Geometry: final body of the model. Coordinates: model frame, mm. Face numbers are marked on the shaded views. A direction names the side the tool comes from. Coordinates: 2 decimals unless noted, no trailing zeros. Order: outer loops, then holes, each group sorted by start corner. A loop starts at its lowest first (then second) coordinate and runs counter-clockwise, first axis right, second up. Notation, with made-up numbers: (-28, 68.5) -> (2, 68.5) arc R15 ccw to (2, 77.5) -> close; hole circle Ø10 at (64, 35). An arc over 180 degrees is marked (long way). Use one line per item in the form item = value.
Autodesk Inventor part; units mm, degrees
ref_plane "YZ Plane" through (0, 0, 0) normal (1, 0, 0) x (0, 1, 0)
ref_plane "XZ Plane" through (0, 0, 0) normal (0, 1, 0) x (-1, 0, 0)
ref_plane "XY Plane" through (0, 0, 0) normal (0, 0, 1) x (1, 0, 0)
sketch "Sketch1" plane through (0, 0, 0) normal (0, 0, 1) x (1, 0, 0)
  point P0 (0, 0)
sketch "Sketch2" plane through (0, 0, 0) normal (0, 1, 0) x (-1, 0, 0)
  arc A0 (-30.6952, -7.0747) -> (-30.6952, 7.0747) centre (0, 0) ccw
  line L0 (-30.6952, 7.0747) -> (-30.6952, -7.0747)
  dimension "d0" = 63
extrude "Extrusion1" add sketch "Sketch2" along normal blind 27
sketch "Sketch3" plane through (0, 27, 0) normal (0, 1, 0) x (0, 0, 1)
  point P0 (0, 0)
  point P1 (0, 0)
hole "Hole1" at (0, 27, 0) direction (0, -1, 0) diameter 58.5 depth 26
sketch "Sketch4" plane through (0, 0, 0) normal (0, -1, 0) x (0, 0, 1)
  circle A0 centre (0, 0) radius 30
  dimension "d11" = 60
extrude "Extrusion2" add sketch "Sketch4" along normal blind 5
sketch "Sketch5" plane through (0, -5, 0) normal (0, -1, 0) x (1, 0, 0)
  point P0 (0, 0)
  point P1 (0, 0)
hole "Hole2" at (0, -5, 0) direction (0, 1, 0) diameter 51.8 depth 11
sketch "Sketch6" plane through (30.6952, 0, 7.0747) normal (1, 0, 0) x (0, 0, -1)
  circle A0 centre (6.9063, 13.867) radius 6.5
  point P0 (7.0747, 0)
  dimension "d23" = 13
extrude "Extrusion3" add sketch "Sketch6" along normal blind 5
sketch "Sketch7" plane through (35.6952, 13.867, 0.1684) normal (1, 0, 0) x (0, 0, -1)
  point P0 (0.1684, -13.867)
  point P1 (0.2284, -0.2272)
hole "Hole3" at (35.6952, 13.6397, -0.06) direction (-1, 0, 0) diameter 4.1 depth 10
properties part number "microscope_holder"
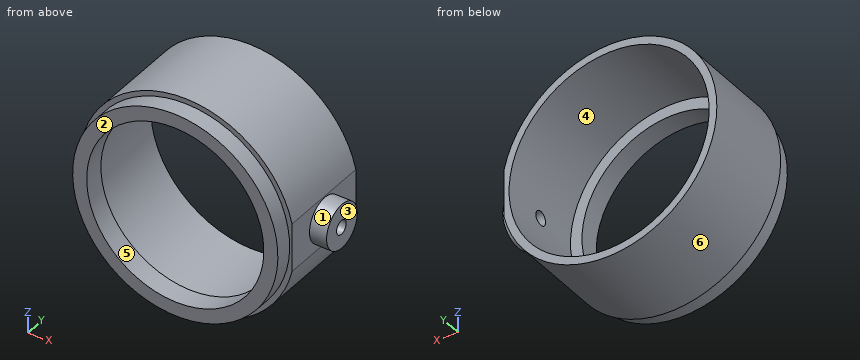
1) Contact query for flat-ended pins moving along their axis: P1, Ø10, axis at x = 12.5, y = 23, coming from the +Z side; P2, Ø1, axis at y = 16.5, z = -1.5, coming from the -X side; P3, Ø3.5, axis at y = 13.64, z = -0.06, coming from the +X side; P4, Ø18.5, axis at x = 12.5, z = 5, coming from the -Y side. Output: stop coordinate, or through.
Results found:
P1 = 30.59
P2 = -31.48
P3 = -29.19
P4 = through
2) Section D-D, the plane x = 17.5. Output: boundary loops of the cut face in (y, z), and give its area (3 significant figures).
Results found:
outline = (-5, -24.37) -> (0, -24.37) -> (0, -26.19) -> (27, -26.19) -> (27, -23.44) -> (1, -23.44) -> (1, -19.09) -> (-5, -19.09) -> close; (-5, 19.09) -> (1, 19.09) -> (1, 23.44) -> (27, 23.44) -> (27, 26.19) -> (0, 26.19) -> (0, 24.37) -> (-5, 24.37) -> close
area = 210 mm2
3) Section C-C, the plane y = 6.5. Output: boundary loops of the cut face in (x, z), and give its area (3 significant figures).
Results found:
outline = (30.7, -7.07) -> (30.7, 7.07) arc R31.5 ccw (long way) to start; hole circle Ø58.5 at (0, 0)
area = 422 mm2
4) Access query for the marked faces 1 and 2. Directions: +Z, -Z, +X, -X, +Y, -Y. A direction counts if a zero-diameter tool reaches every point of the face in a straight line with its end or side. Return the directions, or none.
Results found:
face_1 = +X
face_2 = +Z, -Z, +X, -X, -Y
5) Section B-B, the plane z = -0.06. Output: boundary loops of the cut face in (x, y).
Results found:
outline = (-31.5, 0) -> (-30, 0) -> (-30, -5) -> (-25.9, -5) -> (-25.9, 1) -> (-29.25, 1) -> (-29.25, 27) -> (-31.5, 27) -> close; (25.9, -5) -> (30, -5) -> (30, 0) -> (30.7, 0) -> (30.7, 7.37) -> (35.7, 7.37) -> (35.7, 11.59) -> (29.25, 11.59) -> (29.25, 1) -> (25.9, 1) -> close; (29.25, 15.69) -> (35.7, 15.69) -> (35.7, 20.36) -> (30.7, 20.36) -> (30.7, 27) -> (29.25, 27) -> close
6) Material intervals for probe 1 along Z at (x, y) = (0, -3.15); probe 2 along X at (y, z) = (21.25, 0), sorted ascending. Write a range as from..to.
Results found:
probe_1 = -30..-25.9, 25.9..30
probe_2 = -31.5..-29.25, 29.25..30.7
7) Pull-direction query (X, two-part tool) for the marked faces 3, 4, 5 and 6; classes: released by +X, released by -X, zero draft, split by the parting line, or undercut.
Results found:
face_3 = released by +X
face_4 = undercut
face_5 = undercut
face_6 = split by the parting line
8) Section A-A, the plane x = 0. Output: boundary loops of the cut face in (y, z), and give its area (3 significant figures).
Results found:
outline = (-5, -30) -> (0, -30) -> (0, -31.5) -> (27, -31.5) -> (27, -29.25) -> (1, -29.25) -> (1, -25.9) -> (-5, -25.9) -> close; (-5, 25.9) -> (1, 25.9) -> (1, 29.25) -> (27, 29.25) -> (27, 31.5) -> (0, 31.5) -> (0, 30) -> (-5, 30) -> close
area = 169 mm2
